Can you work these out from the drawing? Everything is in mm from the part's minimum corner. A direction names the side the tool comes from. Give positions to 0.01 mm unless a question says otherwise; leave off trailing zeros. Loops run counter-clockwise (first coordinate to the right, second up) from the corner with the lowest first, then second, coordinate; pieces in that order, holes last. Notation, with made-up numbers: (-26, 74.25) - (22, 74.25) arc R35 cw to (22, 107.25) - close; hole circle Ø11 at (76, -23.5). An arc over 180 degrees is marked (long way). One line per item, written item: value. Start each with the question number.
Q1. If we mould it in two halves opening along Z, with no side actions, what happens to the marked faces 3, 4 and 5? For each: released by +Z, released by -Z, zero draft, split by the parting line, or undercut.
Q2. I want a section at A-A (y = 34). Please give me the cut outline in (x, z).
Q3. I want a section at D-D (z = 7). Count the separate pieces of the cut face and the enclosed holes in it, then the cut area to 3 significant figures.
Q4. If I drill on line 1 (Y direction, x = 13.85, z = 1.25) (3 decimals); line 2 (Y direction, x = 13.5, z = 10); line 3 (Y direction, x = 24.5, z = 13.75), over which ranges is the centre line in solid material (lowest first)? Write a range as from..to.
Q5. I want a section at B-B (z = 13.85). Please give me the cut outline in (x, y) (3 decimals).
Q6. I want a section at C-C (x = 13.85). Please give me the cut outline in (y, z) (3 decimals), then the cut area to 3 significant figures.
Q7. For the marked faces 1 and 2, which set-ups out of +Z, -Z, +X, -X, +Y, -Y let a thin tool reach every point of the face, with its end or its side?
Q8. I'm going to push flat-ended pins straight in: P1, Ø2, axis at x = 18.5, z = 20.5, coming from the -Y side; P2, Ø3.5, axis at x = 13.85, y = 30.5, coming from the -Z side. Where does each tip first touch, or does it pass through?
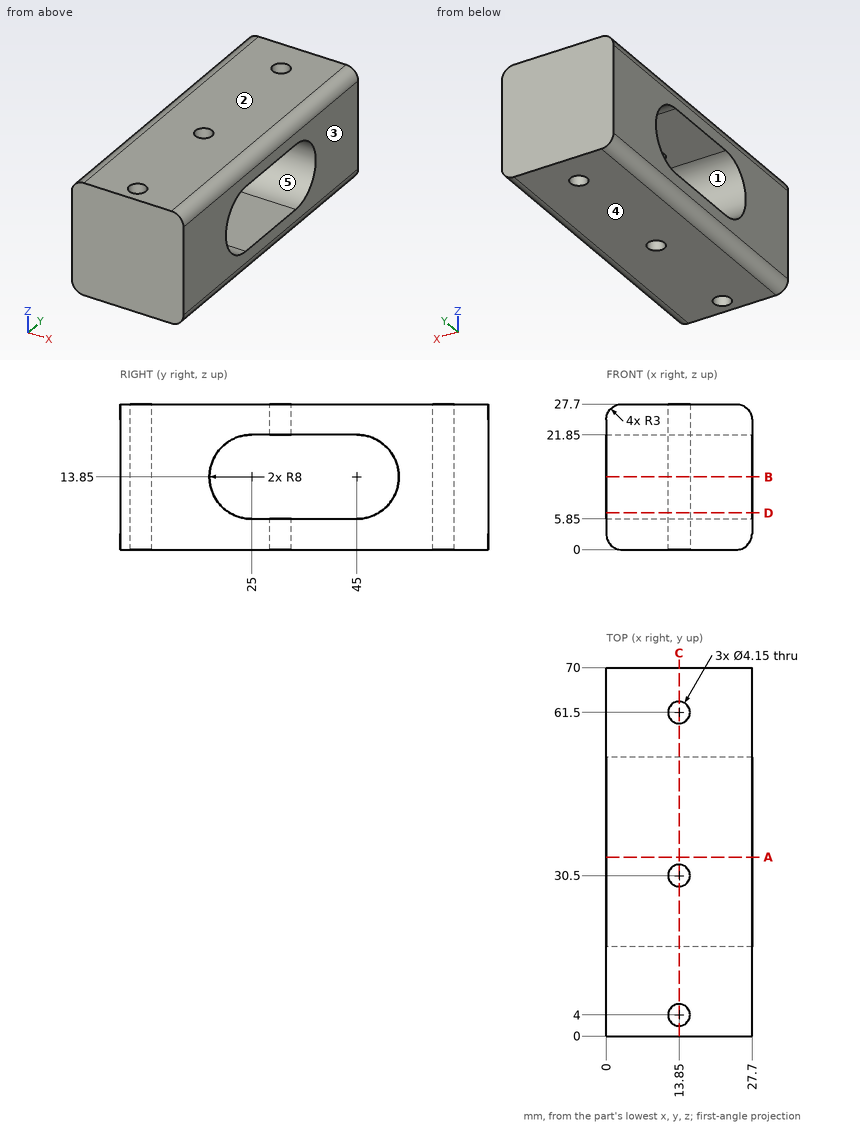
Worked answers:
1. face 3: zero draft
1. face 4: released by -Z
1. face 5: undercut
2. outline: (0, 3) arc R3 ccw to (3, 0) - (24.7, 0) arc R3 ccw to (27.7, 3) - (27.7, 5.85) - (0, 5.85) - close; (0, 21.85) - (27.7, 21.85) - (27.7, 24.7) arc R3 ccw to (24.7, 27.7) - (3, 27.7) arc R3 ccw to (0, 24.7) - close
3. separate pieces: 2
3. enclosed holes: 2
3. area: 1,130 mm²
4. line 1: y = 0..1.925, 6.075..28.425, 32.575..59.425, 63.575..70
4. line 2: y = 0..1.95, 6.05..17.99, 52.01..59.45, 63.55..70
4. line 3: y = 0..17, 53..70
5. outline: (0, 0) - (27.7, 0) - (27.7, 17) - (0, 17) - close; (0, 53) - (27.7, 53) - (27.7, 70) - (0, 70) - close; hole circle Ø4.15 at (13.85, 4); hole circle Ø4.15 at (13.85, 61.5)
6. outline: (0, 0) - (1.925, 0) - (1.925, 27.7) - (0, 27.7) - close; (6.075, 0) - (28.425, 0) - (28.425, 5.85) - (25, 5.85) arc R8 cw to (25, 21.85) - (28.425, 21.85) - (28.425, 27.7) - (6.075, 27.7) - close; (32.575, 0) - (59.425, 0) - (59.425, 27.7) - (32.575, 27.7) - (32.575, 21.85) - (45, 21.85) arc R8 cw to (45, 5.85) - (32.575, 5.85) - close; (63.575, 0) - (70, 0) - (70, 27.7) - (63.575, 27.7) - close
6. area: 1,140 mm²
7. face 1: +X, -X
7. face 2: +Z, +X, -X, +Y, -Y
8. P1: stops at y = 0
8. P2: passes through
